Autodesk Inventor part; units mm, degrees
ref_plane "YZ Plane" through (0, 0, 0) normal (1, 0, 0) x (0, 1, 0)
ref_plane "XZ Plane" through (0, 0, 0) normal (0, 1, 0) x (-1, 0, 0)
ref_plane "XY Plane" through (0, 0, 0) normal (0, 0, 1) x (1, 0, 0)
sketch "Boceto2" plane through (0, 0, 0) normal (0, 1, 0) x (-1, 0, 0)
  line L0 (7.5, 100) -> (-7.5, 100)
  line L1 (-7.5, 100) -> (-7.5, -100)
  line L2 (-7.5, -100) -> (7.5, -100)
  line L3 (7.5, -100) -> (7.5, 100)
  line L4 (7.5, 100) -> (-7.5, -100) construction
  line L5 (-7.5, 100) -> (7.5, -100) construction
  point P0 (0, 0)
  dimension "d7" = 15
  dimension "d8" = 200
extrude "Extrusión1" add sketch "Boceto2" along normal blind 10
sketch "Boceto3" plane through (0, 10, 0) normal (0, 1, 0) x (1, 0, 0)
  circle A0 centre (3.25, 58.25) radius 1.75
  line L0 (5, 50) -> (-5, 50)
  line L1 (-5, 50) -> (-5, 60)
  line L2 (-5, 60) -> (5, 60)
  line L3 (5, 60) -> (5, 50)
  line L4 (5, 50) -> (-5, 60) construction
  line L5 (-5, 50) -> (5, 60) construction
  circle A1 centre (-3.25, 51.75) radius 1.75
  line L6 (7.5, 100) -> (-7.5, 100)
  line L7 (-7.5, 0) -> (3.408, 0)
  line L8 (5, -60) -> (5, -50)
  line L9 (-5, -60) -> (5, -60)
  line L10 (5, -50) -> (-5, -50)
  line L11 (-5, -50) -> (-5, -60)
  line L12 (-5, -50) -> (5, -60) construction
  circle A2 centre (-3.25, -51.75) radius 1.75
  line L13 (5, -50) -> (-5, -60) construction
  circle A3 centre (3.25, -58.25) radius 1.75
  line L14 (-7.5, -100) -> (7.5, -100)
  point P0 (0, 0)
  point P1 (-5, 55)
  point P2 (0, 100)
  point P3 (-5, -55)
  dimension "d11" = 3.5
  dimension "d12" = 1.75
  dimension "d13" = 1.75
  dimension "d14" = 1.75
  dimension "d15" = 1.75
  dimension "d16" = 10
  dimension "d17" = 10
  dimension "d19" = 40
  dimension "d81" = 40
hole "Agujero1" at (3.25, 10, 58.25) at (-3.25, 10, 51.75) at (3.25, 10, -58.25) at (-3.25, 10, -51.75) direction (0, -1, 0) diameter 3.5 end through all
sketch "Boceto4" plane through (0, 10, 0) normal (0, 1, 0) x (1, 0, 0)
  line L0 (-7.5, 100) -> (-7.5, -100)
  line L1 (-7.5, -100) -> (7.5, -100)
  line L2 (7.5, -100) -> (7.5, -80)
  line L3 (7.5, -80) -> (-7.5, -80)
  line L4 (-7.5, -80) -> (-7.5, -100)
  line L5 (-7.5, 0) -> (1.0116, 0)
  line L6 (-7.5, -100) -> (-7.5, 100)
  line L7 (-7.5, 100) -> (7.5, 100)
  line L8 (7.5, 100) -> (7.5, 80)
  line L9 (7.5, 80) -> (-7.5, 80)
  line L10 (-7.5, 80) -> (-7.5, 100)
  point P0 (0, 0)
  point P1 (-7.5, -80)
  point P2 (-7.5, 80)
  dimension "d27" = 15
  dimension "d28" = 20
extrude "Extrusión2" add sketch "Boceto4" along normal blind 80
sketch "Boceto5" plane through (0, 90, 0) normal (0, 1, 0) x (1, 0, 0)
  line L0 (-7.5, -100) -> (7.5, -100)
  line L1 (-7.5, -100) -> (49.5, -100)
  line L2 (49.5, -100) -> (49.5, 100)
  line L3 (49.5, 100) -> (-7.5, 100)
  line L4 (-7.5, 100) -> (-7.5, -100)
  line L5 (49.5, -100) -> (-150.5, -100)
  line L6 (-150.5, -100) -> (-150.5, 100)
  line L7 (-150.5, 100) -> (49.5, 100)
  line L8 (49.5, 100) -> (49.5, -100)
  point P0 (0, 0)
  point P1 (-7.5, 100)
  dimension "d31" = 57
  dimension "d32" = 200
  dimension "d75" = 200
extrude "Extrusión3" add sketch "Boceto5" along normal blind 110
sketch "Boceto6" plane through (0, 200, 0) normal (0, 1, 0) x (1, 0, 0)
  line L0 (49.5, 100) -> (7.5, 100)
  line L1 (49.5, 100) -> (29.5, 100)
  line L2 (29.5, 100) -> (29.5, 80)
  line L3 (7.5, -100) -> (49.5, -100)
  line L4 (28.5, -100) -> (28.5, -80)
  line L5 (-150.5, 100) -> (-150.5, -100)
  line L6 (29.5, 80) -> (-150.5, 80)
  line L7 (-150.5, 80) -> (-150.5, -80)
  line L8 (-150.5, -80) -> (29.5, -80)
  line L9 (29.5, -80) -> (29.5, 80)
  line L10 (-150.5, -100) -> (49.5, -100)
  point P0 (7.5, 80)
  point P1 (-50.5, -100)
  dimension "d36" = 20
  dimension "d37" = 20
  dimension "d38" = 20
  dimension "d77" = 20
extrude "Extrusión4" cut sketch "Boceto6" against normal blind 90 contours L8 L5 L6 L9
sketch "Boceto7" plane through (-150.5, 90, -100) normal (-1, 0, 0) x (0, 0, 1)
  line L0 (0, 110) -> (20, 110)
  line L1 (20, 110) -> (10, 110)
  line L2 (10, 110) -> (10, 20)
  line L3 (10, 20) -> (20, 20)
  line L4 (20, 20) -> (20, 110)
  line L5 (180, 110) -> (180, 20)
  line L6 (180, 110) -> (190, 110)
  line L7 (190, 110) -> (190, 20)
  line L8 (190, 20) -> (180, 20)
  line L9 (180, 20) -> (180, 110)
  line L10 (200, 0) -> (200, 110)
  line L11 (0, 0) -> (0, 110)
  line L12 (0, 110) -> (10, 110)
  line L13 (10, 110) -> (10, 20)
  line L14 (10, 20) -> (0, 20)
  line L15 (0, 20) -> (0, 110)
  line L16 (200, 110) -> (0, 110)
  line L17 (200, 110) -> (190, 110)
  line L18 (190, 110) -> (190, 20)
  line L19 (190, 20) -> (200, 20)
  line L20 (200, 20) -> (200, 110)
  point P0 (100, -90)
  dimension "d63" = 10
  dimension "d65" = 10
  dimension "d76" = 10
extrude "Extrusión5" cut sketch "Boceto7" against normal blind 30 contours L6 L7 L8 L5 | L0 L4 L3 L2
sketch "Boceto8" plane through (-7.5, 0, 100) normal (0, 0, 1) x (1, 0, 0)
  line L0 (-113, 110) -> (-113, 200)
  line L1 (-113, 200) -> (-113, 110)
  circle A0 centre (-124.75, 183.25) radius 1.75
  line L2 (-123, 175) -> (-133, 175)
  line L3 (-133, 175) -> (-133, 185)
  line L4 (-133, 185) -> (-123, 185)
  line L5 (-123, 185) -> (-123, 175)
  line L6 (-123, 175) -> (-133, 185) construction
  line L7 (-133, 175) -> (-123, 185) construction
  circle A1 centre (-131.25, 176.75) radius 1.75
  line L8 (-143, 200) -> (57, 200)
  line L9 (-143, 90) -> (-143, 200)
  line L10 (-113, 155) -> (-128, 155)
  line L11 (-123, 125) -> (-123, 135)
  line L12 (-133, 125) -> (-123, 125)
  line L13 (-123, 135) -> (-133, 125) construction
  line L14 (-123, 135) -> (-133, 135)
  line L15 (-133, 135) -> (-123, 125) construction
  circle A2 centre (-131.25, 133.25) radius 1.75
  line L16 (-133, 135) -> (-133, 125)
  circle A3 centre (-124.75, 126.75) radius 1.75
  line L17 (-143, 110) -> (-113, 110)
  point P0 (7.5, 0)
  point P1 (-133, 180)
  point P2 (-123, 180)
  point P3 (-133, 130)
  point P4 (-123, 130)
  dimension "d45" = 3.5
  dimension "d46" = 1.75
  dimension "d47" = 1.75
  dimension "d48" = 1.75
  dimension "d49" = 1.75
  dimension "d50" = 10
  dimension "d51" = 10
  dimension "d52" = 15
  dimension "d53" = 10
  dimension "d54" = 10
  dimension "d55" = 15
hole "Agujero2" at (-132.25, 183.25, 100) at (-138.75, 176.75, 100) at (-138.75, 133.25, 100) at (-132.25, 126.75, 100) direction (0, 0, -1) diameter 3.5 end through all
ref_plane "Plano de trabajo1" through (-150.5, 90, 100) normal (0, -1, 0) x (1, 0, 0)
split "Dividir1" plane through (-150.5, 90, 100) removes the side toward (0, -1, 0)
ref_plane "Plano de trabajo2" through (49.5, 90, 0) normal (0, 0, -1) x (-1, 0, 0)
ref_plane "Plano de trabajo3" through (-50.5, 90, 100) normal (1, 0, 0) x (0, 0, -1)
ref_plane "Plano de trabajo4" through (0, 145, 0) normal (0, 1, 0) x (1, 0, 0)
sketch "Boceto9" plane through (-150.5, 90, 100) normal (0, 0, 1) x (1, 0, 0)
  line L0 (85.0357, 30) -> (115.0357, 30)
  circle A0 centre (110.0357, 25) radius 1.75
  line L1 (90.0357, 25) -> (110.0357, 25)
  line L2 (115.0357, 30) -> (115.0357, 20)
  circle A1 centre (90.0357, 25) radius 1.75
  line L3 (85.0357, 20) -> (115.0357, 30) construction
  line L4 (85.0357, 30) -> (115.0357, 20) construction
  line L5 (85.0357, 20) -> (85.0357, 30)
  line L6 (115.0357, 20) -> (85.0357, 20)
  line L7 (200, 0) -> (200, 110)
  line L8 (200, 55) -> (88.2857, 55)
  circle A2 centre (90.0357, 85) radius 1.75
  line L9 (85.0357, 80) -> (115.0357, 80)
  line L10 (85.0357, 80) -> (115.0357, 90) construction
  line L11 (85.0357, 90) -> (85.0357, 80)
  line L12 (115.0357, 90) -> (85.0357, 90)
  line L13 (85.0357, 90) -> (115.0357, 80) construction
  circle A3 centre (110.0357, 85) radius 1.75
  line L14 (90.0357, 85) -> (110.0357, 85)
  line L15 (115.0357, 80) -> (115.0357, 90)
  line L16 (100.0357, 55) -> (185.099, 55) construction
  line L17 (160, 70) -> (160, 40)
  circle A4 centre (165, 45) radius 1.75
  line L18 (170, 40) -> (170, 70)
  line L19 (170, 70) -> (160, 40) construction
  line L20 (160, 40) -> (170, 40)
  line L21 (160, 70) -> (170, 40) construction
  circle A5 centre (165, 65) radius 1.75
  line L22 (165, 65) -> (165, 45)
  line L23 (170, 70) -> (160, 70)
  circle A6 centre (55, 65) radius 1.75
  line L24 (60, 70) -> (60, 40)
  line L25 (60, 40) -> (50, 40)
  circle A7 centre (55, 45) radius 1.75
  line L26 (55, 65) -> (55, 45)
  line L27 (60, 70) -> (50, 40) construction
  line L28 (50, 40) -> (50, 70)
  line L29 (50, 70) -> (60, 40) construction
  line L30 (50, 70) -> (60, 70)
  line L31 (30, 110) -> (30, 20)
  point P0 (150.5, -90)
  point P1 (100.0357, 34.7141)
  point P2 (100.0357, 34.7141)
  point P3 (85.0357, 36.6749)
  point P4 (115.0357, 25)
  point P5 (115.0357, 85)
  point P6 (189.1833, 40)
  point P7 (165, 70)
  point P8 (70.0357, 40)
  point P9 (55, 70)
  dimension "d89" = 10
  dimension "d90" = 30
  dimension "d91" = 5
  dimension "d92" = 5
  dimension "d93" = 5
  dimension "d94" = 5
  dimension "d95" = 30
  dimension "d96" = 5
  dimension "d97" = 5
  dimension "d98" = 3.5
  dimension "d99" = 5
  dimension "d100" = 5
  dimension "d101" = 5
  dimension "d102" = 5
  dimension "d103" = 5
  dimension "d104" = 20
hole "Agujero3" at (-60.4643, 175, 100) at (-40.4643, 175, 100) at (14.5, 155, 100) at (-95.5, 155, 100) at (-95.5, 135, 100) at (-60.4643, 115, 100) at (-40.4643, 115, 100) at (14.5, 135, 100) direction (0, 0, -1) diameter 3.5 end through all
sketch "Boceto10" plane through (49.5, 90, 100) normal (1, 0, 0) x (0, 0, -1)
  line L0 (85.0357, 30) -> (115.0357, 30)
  circle A0 centre (110.0357, 25) radius 1.75
  line L1 (90.0357, 25) -> (110.0357, 25)
  line L2 (115.0357, 30) -> (115.0357, 20)
  circle A1 centre (90.0357, 25) radius 1.75
  line L3 (85.0357, 30) -> (115.0357, 20) construction
  line L4 (85.0357, 20) -> (85.0357, 30)
  line L5 (115.0357, 20) -> (85.0357, 20)
  line L6 (85.0357, 20) -> (115.0357, 30) construction
  line L7 (160, 70) -> (160, 40)
  circle A2 centre (165, 45) radius 1.75
  line L8 (160, 40) -> (170, 40)
  line L9 (165, 65) -> (165, 45)
  circle A3 centre (165, 65) radius 1.75
  line L10 (170, 70) -> (160, 40) construction
  line L11 (170, 70) -> (160, 70)
  line L12 (160, 70) -> (170, 40) construction
  line L13 (170, 40) -> (170, 70)
  line L14 (40, 70) -> (40, 40)
  line L15 (35, 65) -> (35, 45)
  circle A4 centre (35, 65) radius 1.75
  line L16 (40, 40) -> (30, 40)
  line L17 (40, 70) -> (30, 40) construction
  line L18 (30, 70) -> (40, 40) construction
  line L19 (30, 70) -> (40, 70)
  line L20 (30, 40) -> (30, 70)
  circle A5 centre (35, 45) radius 1.75
  circle A6 centre (90.0357, 85) radius 1.75
  line L21 (85.0357, 80) -> (115.0357, 80)
  line L22 (115.0357, 80) -> (115.0357, 90)
  circle A7 centre (110.0357, 85) radius 1.75
  line L23 (90.0357, 85) -> (110.0357, 85)
  line L24 (85.0357, 80) -> (115.0357, 90) construction
  line L25 (85.0357, 90) -> (85.0357, 80)
  line L26 (115.0357, 90) -> (85.0357, 90)
  line L27 (85.0357, 90) -> (115.0357, 80) construction
  line L28 (0, 0) -> (0, 110)
  line L29 (200, 0) -> (200, 110)
  point P0 (100, -90)
  point P1 (100.0357, 34.7141)
  point P2 (100.0357, 34.7141)
  point P3 (85.0357, 36.6749)
  point P4 (115.0357, 25)
  point P5 (88.2857, 55)
  point P6 (189.1833, 40)
  point P7 (165, 70)
  point P8 (70.0357, 40)
  point P9 (35, 70)
  point P10 (115.0357, 85)
  point P11 (100.0357, 55)
  dimension "d112" = 10
  dimension "d113" = 30
  dimension "d114" = 5
  dimension "d115" = 5
  dimension "d116" = 5
  dimension "d117" = 5
  dimension "d118" = 5
  dimension "d119" = 5
  dimension "d120" = 3.5
  dimension "d121" = 5
  dimension "d122" = 5
  dimension "d123" = 5
  dimension "d124" = 5
  dimension "d125" = 5
  dimension "d126" = 30
  dimension "d127" = 30
hole "Agujero4" at (49.5, 175, 9.9643) at (49.5, 175, -10.0357) at (49.5, 155, 65) at (49.5, 135, 65) at (49.5, 115, 9.9643) at (49.5, 115, -10.0357) at (49.5, 135, -65) at (49.5, 155, -65) direction (-1, 0, 0) diameter 3.5 end through all
split "Dividir2" plane through (-50.5, 90, 100) removes the side toward (-1, 0, 0)
split "Dividir3" plane through (0, 145, 0) removes the side toward (0, -1, 0)
split "Dividir4" plane through (49.5, 90, 0) removes the side toward (0, 0, -1)
properties part number "container_front_head_6"
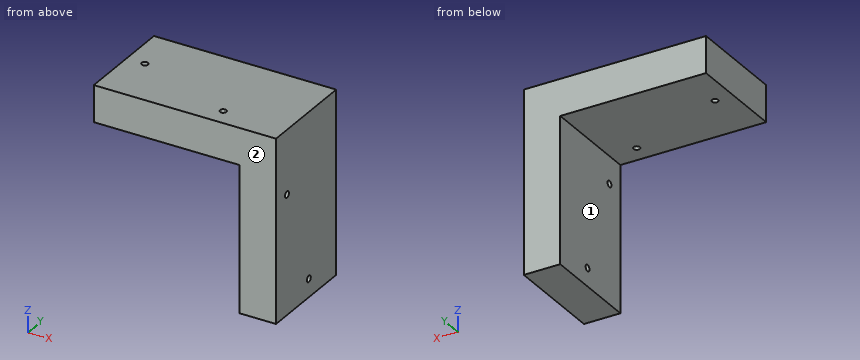
For this review, take the finished solid that the model builds, in its own axes (mm). Face numbers are marked on the shaded views. A direction names the side the tool comes from. Round coordinates to 2 decimals unless told otherwise and drop trailing zeros. Loops run counter-clockwise (first coordinate to the right, second up) from the corner with the lowest first, then second, coordinate; pieces in that order, holes last. Notation, with made-up numbers: (-40, -28) - (-2, -28) arc R15 cw to (-2, -19) - close; hole circle Ø11 at (81.5, -35). An arc over 180 degrees is marked (long way). One line per question, with ' | ' between items.
Q1. Take a section at A-A (z = 65). Give the boundary of the cut face in (x, y).
Taken from the geometry:
outline: (29.5, 145) - (49.5, 145) - (49.5, 153.25) - (29.5, 153.25) - close; (29.5, 156.75) - (49.5, 156.75) - (49.5, 200) - (29.5, 200) - close
Q2. For pin 1 (4 mm diameter, centred on x = -40.46, y = 175, fed in from -Z); pin 2 (5.5 mm diameter, centred on y = 155, z = 65, fed in from +X); pin 3 (10 mm diameter, centred on y = 159.5, z = 54.5, fed in from -X), all flat-tipped, find the tip position at first contact; note any pin that passes through.
Taken from the geometry:
pin 1: stops at z = 80 | pin 2: stops at x = 49.5 | pin 3: stops at x = 29.5
Q3. For line 1 along X through (y, z) = (155, 91); line 2 along X through (y, z) = (175, 84); line 3 along Z through (x, y) = (42, 155), list the stretches that pass through material, from the lowest coordinate up. Write a range as [from, to].
Taken from the geometry:
line 1: x = [-50.5, 12.75], [16.25, 49.5] | line 2: x = [-50.5, -42.21], [-38.71, 49.5] | line 3: z = [0, 63.25], [66.75, 100]
Q4. Take a section at B-B (x = 14.5). Give the boundary of the cut face in (y, z).
Taken from the geometry:
outline: (145, 80) - (153.25, 80) - (153.25, 100) - (145, 100) - close; (156.75, 80) - (200, 80) - (200, 100) - (156.75, 100) - close
Q5. Take a section at C-C (y = 175). Give the boundary of the cut face in (x, z), and give its area (3 significant figures).
Taken from the geometry:
outline: (-50.5, 80) - (-42.21, 80) - (-42.21, 100) - (-50.5, 100) - close; (-38.71, 80) - (29.5, 80) - (29.5, 11.71) - (49.5, 11.71) - (49.5, 100) - (-38.71, 100) - close; (29.5, 0) - (49.5, 0) - (49.5, 8.21) - (29.5, 8.21) - close | area: 3,460 mm²
Q6. Tool access review of the marked faces 1 and 2: name each direction out of +Z, -Z, +X, -X, +Y, -Y from which nothing blocks a thin tool from reaching the whole face with its end or side.
Taken from the geometry:
face 1: -Z, -X, +Y, -Y | face 2: +Z, -Z, +X, -X, -Y
